Source: CAD feature listing. Evaluate the final solid. Frame: model axes, mm. Give positions to 0.01 mm unless a question says otherwise; leave off trailing zeros. Write each loop counter-clockwise with the first axis right and the second up, starting at its lowest first coordinate (ties: lowest second). Pieces come first, ordered by that corner, then holes. Notation, with made-up numbers: (81, 5.25) - (109, 5.25) arc R34 cw to (109, 38.25) - close; hole circle Ø11 at (17, -8.75). An arc over 180 degrees is marked (long way). Answer as a JSON object with one key per item and string values. Group by question number.
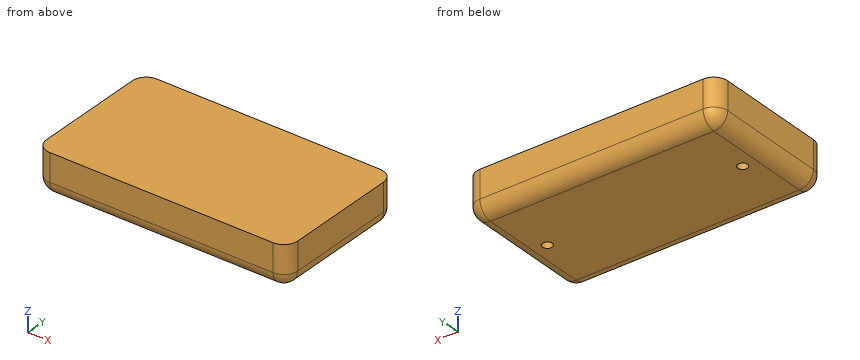
from build123d import *

# Parameters (mm, degrees)
F0_W     = 90
F0_H     = 50
F1_DEPTH = 10
F2_W     = 90
F2_H     = 50
F3_DEPTH = 2.5
F4_W     = 90
F4_H     = 50
F5_DEPTH = 2.5
F6_R     = 5
F7_R     = 5
F9_DEPTH = 12.5


with BuildPart() as f1:
    # F0 (on Top) → F1 (new body)
    with BuildSketch(Plane.XY):
        Rectangle(F0_W, F0_H)
        Polygon((-28.1291651246, -2.75), (-16.8708348754, -2.75), (-11.2416697508, -12.5), (-16.8708348754, -22.25), (-28.1291651246, -22.25), (-33.7583302492, -12.5), align=None, mode=Mode.SUBTRACT)
        Polygon((16.8708348754, -2.75), (28.1291651246, -2.75), (33.7583302492, -12.5), (28.1291651246, -22.25), (16.8708348754, -22.25), (11.2416697508, -12.5), align=None, mode=Mode.SUBTRACT)
        Polygon((-28.1291651246, 22.25), (-16.8708348754, 22.25), (-11.2416697508, 12.5), (-16.8708348754, 2.75), (-28.1291651246, 2.75), (-33.7583302492, 12.5), align=None, mode=Mode.SUBTRACT)
        Polygon((11.2416697508, 12.5), (16.8708348754, 22.25), (28.1291651246, 22.25), (33.7583302492, 12.5), (28.1291651246, 2.75), (16.8708348754, 2.75), align=None, mode=Mode.SUBTRACT)
    extrude(amount=F1_DEPTH)

    # F2 (on face) → F3 (join)
    with BuildSketch(Plane.XY.offset(10)):
        Rectangle(F2_W, F2_H)
    extrude(amount=F3_DEPTH)

    # F4 (on face) → F5 (join)
    with BuildSketch(Plane(origin=(0, 0, 0), x_dir=(1, 0, 0), z_dir=(0, 0, -1))):
        Rectangle(F4_W, F4_H)
    extrude(amount=F5_DEPTH)

    # F6
    f6_edges = [f1.edges().sort_by_distance(p)[0] for p in [
        (-45, 25, 5),
        (45, 25, 5),
        (45, -25, 5),
        (-45, -25, 5),
    ]]
    fillet(f6_edges, radius=F6_R)

    # F7
    f7_edges = [f1.edges().sort_by_distance(p)[0] for p in [
        (0, -25, -2.5),
        (43.535534, -23.535534, -2.5),
        (45, 0, -2.5),
        (43.535534, 23.535534, -2.5),
        (0, 25, -2.5),
        (-45, 0, -2.5),
        (-43.535534, 23.535534, -2.5),
        (-43.535534, -23.535534, -2.5),
    ]]
    fillet(f7_edges, radius=F7_R)

    # F8 (on face) → F9 (cut)
    with BuildSketch(Plane(origin=(0, 0, -2.5), x_dir=(1, 0, 0), z_dir=(0, 0, -1))):
        with BuildLine():
            Line((-33.25, 0), (-35, 0))
            Line((-35, 0), (-36.75, 0))
            ThreePointArc((-36.75, 0), (-35, -1.75), (-33.25, 0))
        make_face()
        with BuildLine():
            Line((-36.75, 0), (-35, 0))
            Line((-35, 0), (-33.25, 0))
            ThreePointArc((-33.25, 0), (-35, 1.75), (-36.75, 0))
        make_face()
        with BuildLine():
            Line((35, 0), (33.25, 0))
            ThreePointArc((33.25, 0), (35, -1.75), (36.75, 0))
            Line((36.75, 0), (35, 0))
        make_face()
        with BuildLine():
            ThreePointArc((36.75, 0), (35, 1.75), (33.25, 0))
            Line((33.25, 0), (35, 0))
            Line((35, 0), (36.75, 0))
        make_face()
    extrude(amount=-F9_DEPTH, mode=Mode.SUBTRACT)


solid = f1.part
Q1. Section B-B on x = 32. Return the cut outline in (y, z).
Q2. Ray query, probe 1 along X at (y, z) = (0, 6.25); probe 2 along Y at (x, z) = (-18, 6.25); probe 3 along Z at (x, y) = (-24, -8.5). Return the intervals inside material, ascending. Write a range as [from, to].
Q3. First-contact query: pin 1 Ø1.5 at (y, z) = (-5, -1) entering from +X; pin 2 Ø1 at (x, z) = (-26.5, 1) entering from +Y. Flat tips, straight axial feed; report the tip coordinate or a pass-through.
Q4. Section D-D on x = -35. Return the cut outline in (y, z).
Q5. Section C-C on y = -9. Return the cut outline in (x, z).
Q6. Section A-A on y = 0. Return the cut outline in (x, z).
Taken from the geometry:
{
 "1": {"outline": "(-25, 2.5) arc R5 ccw to (-20, -2.5) - (20, -2.5) arc R5 ccw to (25, 2.5) - (25, 12.5) - (-25, 12.5) - close; hole (-15.55, 0) - (-9.45, 0) - (-9.45, 10) - (-15.55, 10) - close; hole (9.45, 0) - (15.55, 0) - (15.55, 10) - (9.45, 10) - close"},
 "2": {"probe 1": "x = [-45, -36.75], [-33.25, 33.25], [36.75, 45]", "probe 2": "y = [-25, -22.25], [-2.75, 2.75], [22.25, 25]", "probe 3": "z = [-2.5, 0], [10, 12.5]"},
 "3": {"pin 1": "stops at x = 44.18", "pin 2": "stops at y = 24.9"},
 "4": {"outline": "(-25, 2.5) arc R5 ccw to (-20, -2.5) - (-1.75, -2.5) - (-1.75, 10) - (1.75, 10) - (1.75, -2.5) - (20, -2.5) arc R5 ccw to (25, 2.5) - (25, 12.5) - (-25, 12.5) - close"},
 "5": {"outline": "(-45, 2.5) arc R5 ccw to (-40, -2.5) - (40, -2.5) arc R5 ccw to (45, 2.5) - (45, 12.5) - (-45, 12.5) - close; hole (-31.74, 0) - (-13.26, 0) - (-13.26, 10) - (-31.74, 10) - close; hole (13.26, 0) - (31.74, 0) - (31.74, 10) - (13.26, 10) - close"},
 "6": {"outline": "(-45, 2.5) arc R5 ccw to (-40, -2.5) - (-36.75, -2.5) - (-36.75, 10) - (-33.25, 10) - (-33.25, -2.5) - (33.25, -2.5) - (33.25, 10) - (36.75, 10) - (36.75, -2.5) - (40, -2.5) arc R5 ccw to (45, 2.5) - (45, 12.5) - (-45, 12.5) - close"}
}
